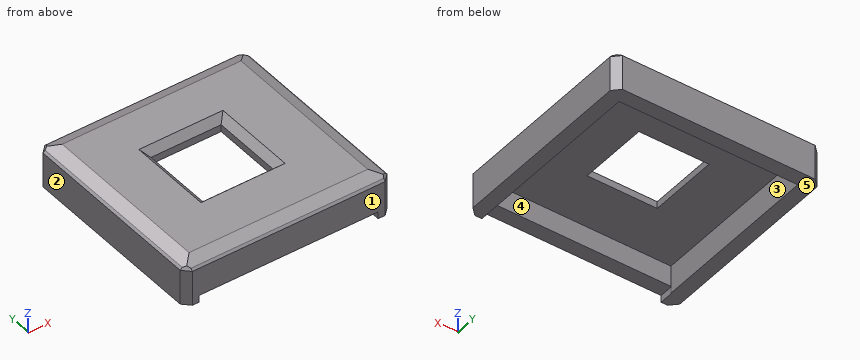
Autodesk Inventor part; units mm, degrees
ref_plane "YZ Plane" through (0, 0, 0) normal (1, 0, 0) x (0, 1, 0)
ref_plane "XZ Plane" through (0, 0, 0) normal (0, 1, 0) x (-1, 0, 0)
ref_plane "XY Plane" through (0, 0, 0) normal (0, 0, 1) x (1, 0, 0)
sketch "Skizze1" plane through (0, 0, 0) normal (0, 0, 1) x (1, 0, 0)
  line L0 (-7.9625, 6.5659) -> (17.5375, 6.5659)
  line L1 (17.5375, 6.5659) -> (17.5375, -17.9341)
  line L2 (17.5375, -17.9341) -> (-7.9625, -17.9341)
  line L3 (-7.9625, -17.9341) -> (-7.9625, 6.5659)
  line L4 (-9.9625, 8.5659) -> (19.5375, 8.5659)
  line L5 (19.5375, 8.5659) -> (19.5375, -19.9341)
  line L6 (19.5375, -19.9341) -> (-9.9625, -19.9341)
  line L7 (-9.9625, -19.9341) -> (-9.9625, 8.5659)
  point P0 (0, 0)
  dimension "d0" = 25.5
  dimension "d1" = 24.5
  dimension "d2" = 2
  dimension "d3" = 2
  dimension "d4" = 2
  dimension "d5" = 2
extrude "Extrusion1" add sketch "Skizze1" along normal blind 4
sketch "Skizze2" plane through (0, 0, 4) normal (0, 0, 1) x (1, 0, 0)
  line L0 (-9.9625, -19.9341) -> (19.5375, -19.9341)
  line L1 (-9.9625, 8.5659) -> (19.5375, 8.5659)
  line L2 (19.5375, 8.5659) -> (19.5375, -19.9341)
  line L3 (19.5375, -19.9341) -> (-9.9625, -19.9341)
  line L4 (-9.9625, -19.9341) -> (-9.9625, 8.5659)
  point P0 (0, 0)
extrude "Extrusion2" add sketch "Skizze2" along normal blind 2
chamfer "Fase1" distance 1 angle 45 8 edges at (4.7875, 8.5659, 6) (-9.9625, -5.6841, 6) (-9.9625, 8.5659, 3) (19.5375, 8.5659, 3) (19.5375, -5.6841, 6) (4.7875, -19.9341, 6) (19.5375, -19.9341, 3) (-9.9625, -19.9341, 3)
chamfer "Fase2" distance 1 angle 45 4 edges at (18.5375, -5.6841, 6) (4.7875, 7.5659, 6) (-8.9625, -5.6841, 6) (4.7875, -18.9341, 6)
sketch "Skizze3" plane through (0, 0, 4) normal (0, 0, -1) x (-1, 0, 0)
  line L0 (-9.5375, -0.4341) -> (0.4625, -0.4341)
  line L1 (0.4625, -0.4341) -> (0.4625, -10.4341)
  line L2 (0.4625, -10.4341) -> (-9.5375, -10.4341)
  line L3 (-9.5375, -10.4341) -> (-9.5375, -0.4341)
  line L4 (-17.5375, 6.5659) -> (7.9625, 6.5659)
  line L5 (7.9625, -17.9341) -> (7.9625, 6.5659)
  line L6 (-17.5375, 6.5659) -> (-17.5375, -17.9341)
  line L7 (-17.5375, -17.9341) -> (7.9625, -17.9341)
  point P0 (0, 0)
  dimension "d16" = 10
  dimension "d17" = 10
  dimension "d18" = 7
  dimension "d19" = 7.5
  dimension "d20" = 8
  dimension "d21" = 7.5
extrude "Extrusion3" cut sketch "Skizze3" against normal blind 67 contours L0 L1 L2 L3
chamfer "Fase3" distance 1 angle 45 4 edges at (4.5375, -0.4341, 6) (-0.4625, -5.4341, 6) (9.5375, -5.4341, 6) (4.5375, -10.4341, 6)
sketch "Skizze4" plane through (0, 0, 0) normal (0, 0, -1) x (-1, 0, 0)
  line L0 (-17.5375, -17.9341) -> (7.9625, -17.9341)
  line L1 (-17.5375, -17.9341) -> (8.0395, -17.9341)
  line L2 (8.0395, -17.9341) -> (8.0395, -21.0501)
  line L3 (8.0395, -21.0501) -> (-17.5375, -21.0501)
  line L4 (-17.5375, -21.0501) -> (-17.5375, -17.9341)
  point P0 (0, 0)
extrude "Extrusion4" cut sketch "Skizze4" against normal blind 1
sketch "Skizze5" plane through (19.5375, -18.9341, 0) normal (1, 0, 0) x (0, 0, -1)
  point P0 (0, 18.9341)
properties part number "Raspberrycamhalter oberteil"
Verification items for the finished model (mm, model axes). Face numbers are marked on the shaded views. A direction names the side the tool comes from. Give positions to 0.01 mm unless a question says otherwise; leave off trailing zeros. Loops run counter-clockwise (first coordinate to the right, second up) from the corner with the lowest first, then second, coordinate; pieces in that order, holes last.
1. Go/stop test with flat-tipped pins: pin 1 Ø2 at (x, y) = (2, 0.5) entering from -Z; pin 2 Ø0.6 at (x, y) = (10, -19.5) entering from -Z. Record where each tip stops, or that it passes through.
2. Section check A-A, the plane z = 3. Enter the section's corners in (x, y).
3. Section check C-C, the plane x = -3.25. Enter the section's corners in (y, z), then the cut area to 3 significant figures.
4. Section check D-D, the plane y = 4.25. Enter the section's corners in (x, z).
5. Section check B-B, the plane y = -1.25. Enter the section's corners in (x, z), then the cut area to 3 significant figures.
6. Mould release check, pull along Y, two halves, no side actions. Record for the marked faces 1, 2 and 3: released by +Y, released by -Y, zero draft, split by the parting line, or undercut.
7. Set-up check for the marked faces 4 and 5: record each of +Z, -Z, +X, -X, +Y, -Y from which the full face is reachable in a straight line by a thin tool's end or side.
8. Thickness scan on line 1 (Y direction, x = 15, z = 3.5); line 2 (X direction, y = 4.25, z = 2); line 3 (Y direction, x = -6.5, z = 0.5). Record the ranges inside material, lowest first.
Geometry says:
1. pin 1: stops at z = 4
1. pin 2: stops at z = 1
2. outline: (-9.96, -18.93) - (-8.96, -19.93) - (18.54, -19.93) - (19.54, -18.93) - (19.54, 7.57) - (18.54, 8.57) - (-8.96, 8.57) - (-9.96, 7.57) - close; hole (-7.96, -17.93) - (17.54, -17.93) - (17.54, 6.57) - (-7.96, 6.57) - close
3. outline: (-19.93, 1) - (-17.93, 1) - (-17.93, 4) - (6.57, 4) - (6.57, 0) - (8.57, 0) - (8.57, 5) - (8.27, 5.29) - (6.57, 6) - (-17.93, 6) - (-19.64, 5.29) - (-19.93, 5) - close
3. area: 69.3 mm2
4. outline: (-9.96, 0) - (-7.96, 0) - (-7.96, 4) - (17.54, 4) - (17.54, 0) - (19.54, 0) - (19.54, 5) - (19.24, 5.29) - (17.54, 6) - (-7.96, 6) - (-9.67, 5.29) - (-9.96, 5) - close
5. outline: (-9.96, 0) - (-7.96, 0) - (-7.96, 4) - (-0.46, 4) - (-0.46, 5) - (-1.46, 6) - (-7.96, 6) - (-9.67, 5.29) - (-9.96, 5) - close; (9.54, 4) - (17.54, 4) - (17.54, 0) - (19.54, 0) - (19.54, 5) - (19.24, 5.29) - (17.54, 6) - (10.54, 6) - (9.54, 5) - close
5. area: 52.3 mm2
6. face 1: released by -Y
6. face 2: zero draft
6. face 3: undercut
7. face 4: -Z
7. face 5: -Z, +X, -X, +Y, -Y
8. line 1: y = -19.93 to -17.93, 6.57 to 8.57
8. line 2: x = -9.96 to -7.96, 17.54 to 19.54
8. line 3: y = 6.57 to 8.57
